The drawing under review shows one solid part. Ordinate dimensions are in mm from its lowest x, y, z. Give positions to 0.01 mm unless a question says otherwise; leave off trailing zeros. Order: outer loops, then holes, each group sorted by start corner. A loop starts at its lowest first (then second) coordinate and runs counter-clockwise, first axis right, second up. Notation, with made-up numbers: (6.25, 57.25) - (52.25, 57.25) arc R19 cw to (52.25, 62.25) - close; hole circle Ø4 at (77.5, -0.75). An arc over 180 degrees is marked (long way). Write item = value, one per line. Start each with the question number.
1. Wall thickness on probe 1 along Z at (x, y) = (2.5, 1.5); probe 2 along X at (y, z) = (1.95, 51); probe 3 along Z at (x, y) = (7, 1.5): over which ranges is each line inside the solid? List them lowest first.
2. We need section A-A, the plane y = 0.45. Give the boundary of the cut face in (x, z), and give its area (3 significant figures).
3. For P1, Ø10, axis at x = 47, z = 50, coming from the -Y side, flat-tipped, find the tip position at first contact; note if it passes through.
4. We need section B-B, the plane x = 11.5. Give the boundary of the cut face in (y, z), and give its area (3 significant figures).
5. We need section C-C, the plane x = 49.5. Give the boundary of the cut face in (y, z), and give its area (3 significant figures).
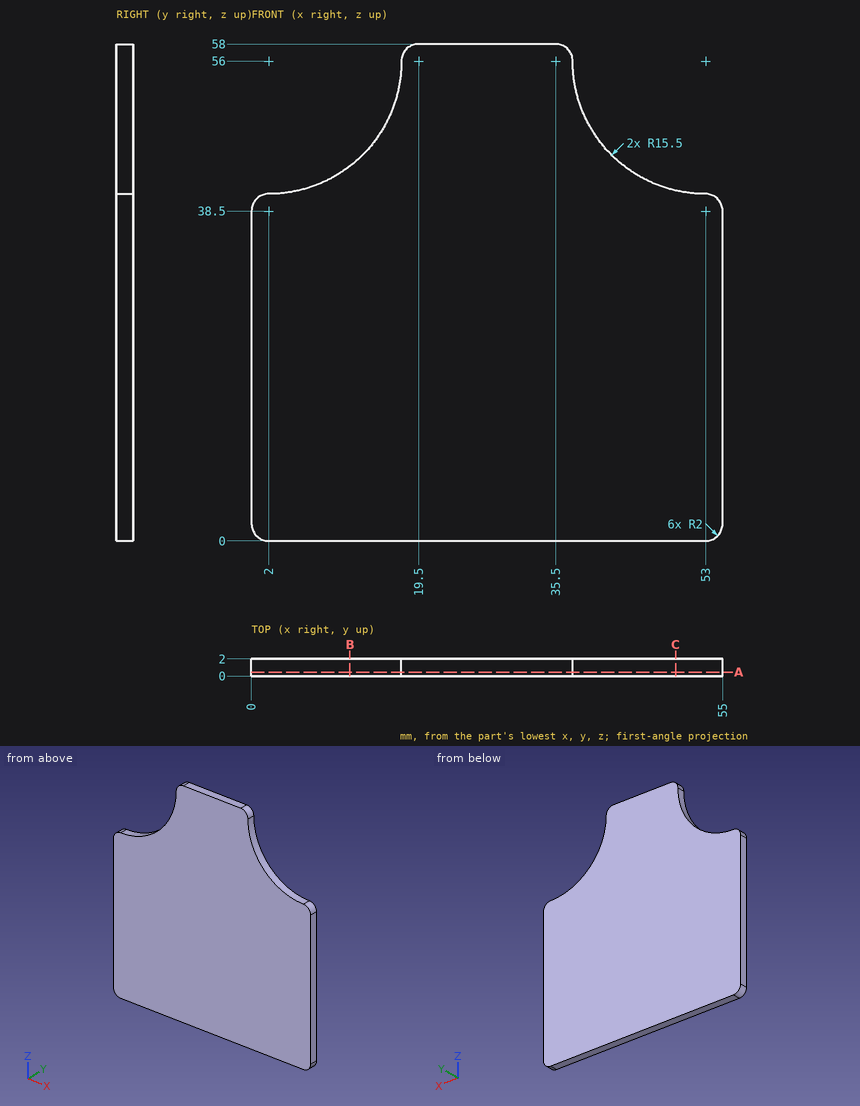
Model answer:
q1.probe_1 = 0 to 40.51
q1.probe_2 = 16.67 to 38.33
q1.probe_3 = 0 to 41.33
q2.outline = (0, 2) arc R2 ccw to (2, 0) - (53, 0) arc R2 ccw to (55, 2) - (55, 38.5) arc R2 ccw to (53, 40.5) arc R15.5 cw to (37.5, 56) arc R2 ccw to (35.5, 58) - (19.5, 58) arc R2 ccw to (17.5, 56) arc R15.5 cw to (2, 40.5) arc R2 ccw to (0, 38.5) - close
q2.area = 2,680 mm2
q3.P1 = through
q4.outline = (0, 0) - (2, 0) - (2, 43.75) - (0, 43.75) - close
q4.area = 87.5 mm2
q5.outline = (0, 0) - (2, 0) - (2, 40.9) - (0, 40.9) - close
q5.area = 81.8 mm2
